```python
from build123d import *

# Parameters (mm, degrees)
F1_DEPTH      = 5
F1_DEPTH_BACK = 5
F2_T1_DEPTH   = 51.4213562373
F2_T3_DEPTH   = 27.589671948


# Not quite as in the source:
# - a fillet or chamfer that OpenCascade refuses, or shapes differently, is made with other operations: its cross-section is extruded or revolved along the edge and cut away or added


with BuildPart() as f1:
    # F0 (on Top) → F1 (new body, two sides)
    with BuildSketch(Plane.XY) as f1_sk:
        with BuildLine():
            ThreePointArc((-7.0367619663, -1.3552663468), (-21.4300874517, -22.6556162733), (-47, -20))
            Line((-47, -20), (-47, -29.3938769134))
            ThreePointArc((-47, -29.3938769134), (-25.6700714676, -32.3872197753), (-7.0367619663, -21.5832515361))
            Line((-7.0367619663, -21.5832515361), (-7.0367619663, -1.3552663468))
        make_face()
        with BuildLine():
            Line((-7.0367619663, 1.3552663468), (-7.0367619663, -1.3552663468))
            ThreePointArc((-7.0367619663, -1.3552663468), (-7, 0), (-7.0367619663, 1.3552663468))
        make_face()
        with BuildLine():
            ThreePointArc((-7.0367619663, 1.3552663468), (-7, 0), (-7.0367619663, -1.3552663468))
            Line((-7.0367619663, -1.3552663468), (-7.0367619663, -21.5832515361))
            ThreePointArc((-7.0367619663, -21.5832515361), (-2.7270271398, -15.2346007472), (0, -8.0622577483))
            ThreePointArc((0, -8.0622577483), (-1, 0), (0, 8.0622577483))
            ThreePointArc((0, 8.0622577483), (-2.7270271398, 15.2346007472), (-7.0367619663, 21.5832515361))
            Line((-7.0367619663, 21.5832515361), (-7.0367619663, 1.3552663468))
        make_face()
        with BuildLine():
            ThreePointArc((-47, 20), (-21.4300874517, 22.6556162733), (-7.0367619663, 1.3552663468))
            Line((-7.0367619663, 1.3552663468), (-7.0367619663, 21.5832515361))
            ThreePointArc((-7.0367619663, 21.5832515361), (-25.6700714676, 32.3872197753), (-47, 29.3938769134))
            Line((-47, 29.3938769134), (-47, 20))
        make_face()
        with BuildLine():
            ThreePointArc((0, -8.0622577483), (-2.7270271398, -15.2346007472), (-7.0367619663, -21.5832515361))
            Line((-7.0367619663, -21.5832515361), (7.0367619663, -21.5832515361))
            ThreePointArc((7.0367619663, -21.5832515361), (2.7270271398, -15.2346007472), (0, -8.0622577483))
        make_face()
        with BuildLine():
            Line((7.0367619663, 21.5832515361), (-7.0367619663, 21.5832515361))
            ThreePointArc((-7.0367619663, 21.5832515361), (-2.7270271398, 15.2346007472), (0, 8.0622577483))
            ThreePointArc((0, 8.0622577483), (2.7270271398, 15.2346007472), (7.0367619663, 21.5832515361))
        make_face()
        with BuildLine():
            ThreePointArc((0, 8.0622577483), (1, 0), (0, -8.0622577483))
            ThreePointArc((0, -8.0622577483), (2.7270271398, -15.2346007472), (7.0367619663, -21.5832515361))
            Line((7.0367619663, -21.5832515361), (7.0367619663, -1.3552663468))
            ThreePointArc((7.0367619663, -1.3552663468), (7, 0), (7.0367619663, 1.3552663468))
            Line((7.0367619663, 1.3552663468), (7.0367619663, 21.5832515361))
            ThreePointArc((7.0367619663, 21.5832515361), (2.7270271398, 15.2346007472), (0, 8.0622577483))
        make_face()
        with BuildLine():
            Line((7.0367619663, -1.3552663468), (7.0367619663, -21.5832515361))
            ThreePointArc((7.0367619663, -21.5832515361), (25.6700714676, -32.3872197753), (47, -29.3938769134))
            Line((47, -29.3938769134), (47, -20))
            ThreePointArc((47, -20), (21.4300874517, -22.6556162733), (7.0367619663, -1.3552663468))
        make_face()
        with BuildLine():
            ThreePointArc((47, 29.3938769134), (25.6700714676, 32.3872197753), (7.0367619663, 21.5832515361))
            Line((7.0367619663, 21.5832515361), (7.0367619663, 1.3552663468))
            ThreePointArc((7.0367619663, 1.3552663468), (21.4300874517, 22.6556162733), (47, 20))
            Line((47, 20), (47, 29.3938769134))
        make_face()
        with BuildLine():
            ThreePointArc((7.0367619663, 1.3552663468), (7, 0), (7.0367619663, -1.3552663468))
            Line((7.0367619663, -1.3552663468), (7.0367619663, 1.3552663468))
        make_face()
        with BuildLine():
            ThreePointArc((0, 8.0622577483), (-1, 0), (0, -8.0622577483))
            ThreePointArc((0, -8.0622577483), (1, 0), (0, 8.0622577483))
        make_face()
    extrude(amount=F1_DEPTH)
    extrude(f1_sk.sketch, amount=-F1_DEPTH_BACK)

    # F2: fillet of radius 5 on 8 edges, made by hand

    # F2_s2 → F2_t1 (cut)
    with BuildSketch(Plane.XY.offset(-25.7106781187)):
        with BuildLine():
            ThreePointArc((-40.3333333333, 23.5702260396), (-44.8867513459, 24.2017883428), (-47, 28.2842712475))
            Line((-47, 28.2842712475), (-47, 20))
            ThreePointArc((-47, 20), (-43.8024463398, 22.0386537791), (-40.3333333333, 23.5702260396))
        make_face()
        with BuildLine():
            ThreePointArc((-40.3333333333, -23.5702260396), (-44.8867513459, -24.2017883428), (-47, -28.2842712475))
            Line((-47, -28.2842712475), (-47, -20))
            ThreePointArc((-47, -20), (-43.8024463398, -22.0386537791), (-40.3333333333, -23.5702260396))
        make_face()
        with BuildLine():
            ThreePointArc((40.3333333333, -23.5702260396), (44.8867513459, -24.2017883428), (47, -28.2842712475))
            Line((47, -28.2842712475), (47, -20))
            ThreePointArc((47, -20), (43.8024463398, -22.0386537791), (40.3333333333, -23.5702260396))
        make_face()
        with BuildLine():
            ThreePointArc((47, 28.2842712475), (44.8867513459, 24.2017883428), (40.3333333333, 23.5702260396))
            ThreePointArc((40.3333333333, 23.5702260396), (43.8024463398, 22.0386537791), (47, 20))
            Line((47, 20), (47, 28.2842712475))
        make_face()
    extrude(amount=F2_T1_DEPTH, mode=Mode.SUBTRACT)

    # F2_s4 → F2_t3 (cut)
    with BuildSketch(Plane.XY.offset(-13.794835974)):
        with BuildLine():
            ThreePointArc((-43.7857142857, -30.8236425293), (-46.1187723552, -28.9881272088), (-47, -26.1533936612))
            Line((-47, -26.1533936612), (-47, -29.3938769134))
            ThreePointArc((-47, -29.3938769134), (-45.4119230492, -30.1516221806), (-43.7857142857, -30.8236425293))
        make_face()
        with BuildLine():
            ThreePointArc((-47, 26.1533936612), (-46.1187723552, 28.9881272088), (-43.7857142857, 30.8236425293))
            ThreePointArc((-43.7857142857, 30.8236425293), (-45.4119230492, 30.1516221806), (-47, 29.3938769134))
            Line((-47, 29.3938769134), (-47, 26.1533936612))
        make_face()
        with BuildLine():
            ThreePointArc((47, -26.1533936612), (46.1187723552, -28.9881272088), (43.7857142857, -30.8236425293))
            ThreePointArc((43.7857142857, -30.8236425293), (45.4119230492, -30.1516221806), (47, -29.3938769134))
            Line((47, -29.3938769134), (47, -26.1533936612))
        make_face()
        with BuildLine():
            ThreePointArc((43.7857142857, 30.8236425293), (46.1187723552, 28.9881272088), (47, 26.1533936612))
            Line((47, 26.1533936612), (47, 29.3938769134))
            ThreePointArc((47, 29.3938769134), (45.4119230492, 30.1516221806), (43.7857142857, 30.8236425293))
        make_face()
    extrude(amount=F2_T3_DEPTH, mode=Mode.SUBTRACT)


solid = f1.part
```
Work out the finished part from the listing and answer in its coordinate system (mm). A direction names the side the tool comes from. Coordinates: 2 decimals unless noted, no trailing zeros. Write each loop counter-clockwise with the first axis right and the second up, starting at its lowest first coordinate (ties: lowest second). Pieces come first, ordered by that corner, then holes.
Q1. Find the intervals of material crossed by line 1 (Y direction, x = -32.5, z = -3.5) (3 decimals); line 2 (Y direction, x = 3.5, z = -2.75); line 3 (X direction, y = 22, z = -0.5), in increasing order.
Q2. A cutting plane is placed at B-B, the plane y = -26. Give the vertices of the cut face in (x, z).
Q3. A cutting plane is placed at A-A, the plane x = 27. Give the vertices of the cut face in (y, z).
Q4. Which of the six approach directions +Z, -Z, +X, -X, +Y, -Y give full straight-line access (tool end or side, diameter ignored) to faces 1 (the face through (0, -21.583, 0)), 2 (the face through (18.396, -20.975, 0.07)), 3 (the face through (7.037, 0, 0)), 4 (the face through (0, 21.583, 0)), 5 (the face through (-7.037, 0, 0))?
Q5. A cutting plane is placed at D-D, the plane x = 2. Give the vertices of the cut face in (y, z), then the cut area to 3 significant figures.
Q6. Each of these flat-tipped pins is pushed along its axis until it touches: pin 1 Ø1.4 at (y, z) = (0, 0.5) entering from +X; pin 2 Ø4 at (y, z) = (-17, -3.5) entering from +X; pin 3 Ø1.5 at (x, z) = (6.5, -2) entering from +Y. Where does it stop, or does it pass through?
Q7. A cutting plane is placed at C-C, the plane z = 3.5. Give the vertices of the cut face in (x, y), then the cut area to 3 significant figures.
Q8. Determine the mould class of faces 6 (the face through (23.679, -31.934, 0.07)), 7 (the face through (-45.8, 29.4, -0.1)), 8 (the face through (0, 3, 5)) for opening direction X: released by +X, released by -X, zero draft, split by the parting line, or undercut.
Findings below:
1. line 1: y = -32.996 to -24.995, 24.995 to 32.996
1. line 2: y = -21.58 to 21.58
1. line 3: x = -20.13 to -7.4, 7.4 to 20.13
2. outline: (-46.45, -5) - (-11.68, -5) - (-11.68, 5) - (-46.45, 5) - close; (11.68, -5) - (46.45, -5) - (46.45, 5) - (11.68, 5) - close
3. outline: (-32.62, -5) - (-24.49, -5) - (-24.49, 5) - (-32.62, 5) - close; (24.49, -5) - (32.62, -5) - (32.62, 5) - (24.49, 5) - close
4. face 1: +Z, -Z, -Y
4. face 2: +Z, -Z
4. face 3: +Z, -Z, +X
4. face 4: +Z, -Z, +Y
4. face 5: +Z, -Z, -X
5. outline: (-21.58, -5) - (21.58, -5) - (21.58, 5) - (-21.58, 5) - close
5. area: 432 mm2
6. pin 1: stops at x = 7.04
6. pin 2: stops at x = 15.75
6. pin 3: stops at y = 21.83
7. outline: (-46.89, -27.22) arc R5 ccw to (-43.79, -30.82) arc R33 ccw to (-7.04, -21.58) - (7.04, -21.58) arc R33 ccw to (43.79, -30.82) arc R5 ccw to (46.89, -27.22) arc R5 ccw to (40.33, -23.57) arc R25 cw to (7.04, -1.36) - (7.04, 1.36) arc R25 cw to (40.33, 23.57) arc R5 ccw to (46.89, 27.22) arc R5 ccw to (43.79, 30.82) arc R33 ccw to (7.04, 21.58) - (-7.04, 21.58) arc R33 ccw to (-43.79, 30.82) arc R5 ccw to (-46.89, 27.22) arc R5 ccw to (-40.33, 23.57) arc R25 cw to (-7.04, 1.36) - (-7.04, -1.36) arc R25 cw to (-40.33, -23.57) arc R5 ccw to start
7. area: 2,030 mm2
8. face 6: undercut
8. face 7: released by -X
8. face 8: zero draft
